The model under review builds one solid part; all positions refer to its coordinate system, in mm. A direction names the side the tool comes from. Round coordinates to 2 decimals unless told otherwise and drop trailing zeros. Order: outer loops, then holes, each group sorted by start corner. A loop starts at its lowest first (then second) coordinate and runs counter-clockwise, first axis right, second up. Notation, with made-up numbers: (-12.5, -20.5) - (38.5, -20.5) arc R25 ccw to (38.5, 4.5) - close; hole circle Ø10 at (5.5, 0). An arc over 180 degrees is marked (long way). One line per question, with ' | ' between items. Start each with the question number.
Item 1: Add section B-B on x = -138.5. State the section outline as (y, z) points, and give its area (3 significant figures).
Item 2: Insertion check: pin 1 Ø2 at (y, z) = (-5.5, -7) entering from -X; pin 2 Ø3 at (x, y) = (-75, -6.5) entering from +Z; pin 3 Ø2 at (x, z) = (91, -5) entering from -Y; pin 4 Ø1.1 at (x, y) = (177.5, -3) entering from +Z. Each pin has a flat end and moves straight along its axis. Give the tip position at first contact, or say it passes through.
Item 3: Add section A-A on x = -46.5. State the section outline as (y, z) points, and give its area (3 significant figures).
Item 4: Draft analysis for pull direction X (two halves, no side actions). For faces 1 (the face through (-2, -5, -22.777)), 2 (the face through (130.237, -5.41, -3.638)), 3 (the face through (172.41, -5.41, -3.82)), state which applies: +X half, -X half, draft (parallel to the pull), parting line (faces both ways), or undercut.
Item 5: For L1, parallel to Z at x = -57.5, y = -1; L2, parallel to Z at x = 127.5, y = -1, list the stretches that pass through material, from the lowest coordinate up. Write a range as [from, to].
Item 6: Tool access review of faces 4 (the face through (177.929, -5, -17)), 5 (the face through (164, -5.4, -3.6)): name each direction out of +Z, -Z, +X, -X, +Y, -Y from which nothing blocks a thin tool from reaching the whole face with its end or side.
from build123d import *

# Parameters (mm, degrees)
F1_DEPTH = 10.9728


with BuildPart() as f1:
    # F0 (on Front) → F1 (new body)
    with BuildSketch(Plane.XZ):
        Polygon((-177.6711943626, -10.0771774247), (-177.6711943626, -22.7771774247), (177.9288056374, -22.7771774247), (177.9288056374, -10.0771774247), (176.5609765906, -10.0771774247), (159.6928365906, -10.0771774247), (159.6916056374, -10.0771774247), (142.8246965906, -10.0771774247), (142.8234656374, -10.0771774247), (125.9565565906, -10.0771774247), (125.9553256374, -10.0771774247), (109.0884165906, -10.0771774247), (109.0871856374, -10.0771774247), (92.2202765906, -10.0771774247), (92.2190456374, -10.0771774247), (75.3521365906, -10.0771774247), (75.3509056374, -10.0771774247), (58.4839965906, -10.0771774247), (58.4827656374, -10.0771774247), (41.6158565906, -10.0771774247), (41.6146256374, -10.0771774247), (24.7477165906, -10.0771774247), (24.7464856374, -10.0771774247), (7.8795765906, -10.0771774247), (7.8783456374, -10.0771774247), (-8.9885634094, -10.0771774247), (-8.9897943626, -10.0771774247), (-25.8567034094, -10.0771774247), (-25.8579343626, -10.0771774247), (-42.7248434094, -10.0771774247), (-42.7260743626, -10.0771774247), (-59.5929834094, -10.0771774247), (-59.5942143626, -10.0771774247), (-76.4611234094, -10.0771774247), (-76.4623543626, -10.0771774247), (-93.3292634094, -10.0771774247), (-93.3304943626, -10.0771774247), (-110.1974034094, -10.0771774247), (-110.1986343626, -10.0771774247), (-127.0655434094, -10.0771774247), (-127.0667743626, -10.0771774247), (-143.9336834094, -10.0771774247), (-143.9349143626, -10.0771774247), (-160.8018234094, -10.0771774247), (-160.8030543626, -10.0771774247), align=None)
        Polygon((-169.2260503769, 2.6228225753), (-177.6711943626, -10.0771774247), (-160.8030543626, -10.0771774247), (-160.8024381229, -10.0762507093), align=None)
        Polygon((-160.8024381229, -10.0762507093), (-160.8030543626, -10.0771774247), (-160.8018234094, -10.0771774247), align=None)
        Polygon((159.6928365906, -10.0771774247), (176.5609765906, -10.0771774247), (168.1367496231, 2.6228225753), (159.6922218771, -10.0762507093), align=None)
        Polygon((-160.8024381229, -10.0762507093), (-160.8018234094, -10.0771774247), (-143.9349143626, -10.0771774247), (-143.9342981229, -10.0762507093), (-152.3579103769, 2.6228225753), align=None)
        Polygon((159.6916056374, -10.0771774247), (159.6928365906, -10.0771774247), (159.6922218771, -10.0762507093), align=None)
        Polygon((-143.9342981229, -10.0762507093), (-143.9349143626, -10.0771774247), (-143.9336834094, -10.0771774247), align=None)
        Polygon((142.8246965906, -10.0771774247), (159.6916056374, -10.0771774247), (159.6922218771, -10.0762507093), (151.2686096231, 2.6228225753), (142.8240818771, -10.0762507093), align=None)
        Polygon((-143.9342981229, -10.0762507093), (-143.9336834094, -10.0771774247), (-127.0667743626, -10.0771774247), (-127.0661581229, -10.0762507093), (-135.4897703769, 2.6228225753), align=None)
        Polygon((142.8234656374, -10.0771774247), (142.8246965906, -10.0771774247), (142.8240818771, -10.0762507093), align=None)
        Polygon((-127.0661581229, -10.0762507093), (-127.0667743626, -10.0771774247), (-127.0655434094, -10.0771774247), align=None)
        Polygon((125.9565565906, -10.0771774247), (142.8234656374, -10.0771774247), (142.8240818771, -10.0762507093), (134.4004696231, 2.6228225753), (125.9559418771, -10.0762507093), align=None)
        Polygon((-127.0661581229, -10.0762507093), (-127.0655434094, -10.0771774247), (-110.1986343626, -10.0771774247), (-110.1980181229, -10.0762507093), (-118.6216303769, 2.6228225753), align=None)
        Polygon((125.9553256374, -10.0771774247), (125.9565565906, -10.0771774247), (125.9559418771, -10.0762507093), align=None)
        Polygon((-110.1980181229, -10.0762507093), (-110.1986343626, -10.0771774247), (-110.1974034094, -10.0771774247), align=None)
        Polygon((109.0884165906, -10.0771774247), (125.9553256374, -10.0771774247), (125.9559418771, -10.0762507093), (117.5323296231, 2.6228225753), (109.0878018771, -10.0762507093), align=None)
        Polygon((-110.1980181229, -10.0762507093), (-110.1974034094, -10.0771774247), (-93.3304943626, -10.0771774247), (-93.3298781229, -10.0762507093), (-101.7534903769, 2.6228225753), align=None)
        Polygon((109.0871856374, -10.0771774247), (109.0884165906, -10.0771774247), (109.0878018771, -10.0762507093), align=None)
        Polygon((-93.3298781229, -10.0762507093), (-93.3304943626, -10.0771774247), (-93.3292634094, -10.0771774247), align=None)
        Polygon((92.2202765906, -10.0771774247), (109.0871856374, -10.0771774247), (109.0878018771, -10.0762507093), (100.6641896231, 2.6228225753), (92.2196618771, -10.0762507093), align=None)
        Polygon((-93.3298781229, -10.0762507093), (-93.3292634094, -10.0771774247), (-76.4623543626, -10.0771774247), (-76.4617381229, -10.0762507093), (-84.8853503769, 2.6228225753), align=None)
        Polygon((92.2190456374, -10.0771774247), (92.2202765906, -10.0771774247), (92.2196618771, -10.0762507093), align=None)
        Polygon((-76.4617381229, -10.0762507093), (-76.4623543626, -10.0771774247), (-76.4611234094, -10.0771774247), align=None)
        Polygon((75.3521365906, -10.0771774247), (92.2190456374, -10.0771774247), (92.2196618771, -10.0762507093), (83.7960496231, 2.6228225753), (75.3515218771, -10.0762507093), align=None)
        Polygon((-76.4617381229, -10.0762507093), (-76.4611234094, -10.0771774247), (-59.5942143626, -10.0771774247), (-59.5935981229, -10.0762507093), (-68.0172103769, 2.6228225753), align=None)
        Polygon((75.3509056374, -10.0771774247), (75.3521365906, -10.0771774247), (75.3515218771, -10.0762507093), align=None)
        Polygon((-59.5935981229, -10.0762507093), (-59.5942143626, -10.0771774247), (-59.5929834094, -10.0771774247), align=None)
        Polygon((58.4839965906, -10.0771774247), (75.3509056374, -10.0771774247), (75.3515218771, -10.0762507093), (66.9279096231, 2.6228225753), (58.4833818771, -10.0762507093), align=None)
        Polygon((-59.5935981229, -10.0762507093), (-59.5929834094, -10.0771774247), (-42.7260743626, -10.0771774247), (-42.7254581229, -10.0762507093), (-51.1490703769, 2.6228225753), align=None)
        Polygon((58.4827656374, -10.0771774247), (58.4839965906, -10.0771774247), (58.4833818771, -10.0762507093), align=None)
        Polygon((-42.7254581229, -10.0762507093), (-42.7260743626, -10.0771774247), (-42.7248434094, -10.0771774247), align=None)
        Polygon((41.6158565906, -10.0771774247), (58.4827656374, -10.0771774247), (58.4833818771, -10.0762507093), (50.0597696231, 2.6228225753), (41.6152418771, -10.0762507093), align=None)
        Polygon((-42.7254581229, -10.0762507093), (-42.7248434094, -10.0771774247), (-25.8579343626, -10.0771774247), (-25.8573181229, -10.0762507093), (-34.2809303769, 2.6228225753), align=None)
        Polygon((41.6146256374, -10.0771774247), (41.6158565906, -10.0771774247), (41.6152418771, -10.0762507093), align=None)
        Polygon((-25.8573181229, -10.0762507093), (-25.8579343626, -10.0771774247), (-25.8567034094, -10.0771774247), align=None)
        Polygon((24.7477165906, -10.0771774247), (41.6146256374, -10.0771774247), (41.6152418771, -10.0762507093), (33.1916296231, 2.6228225753), (24.7471018771, -10.0762507093), align=None)
        Polygon((-25.8573181229, -10.0762507093), (-25.8567034094, -10.0771774247), (-8.9897943626, -10.0771774247), (-8.9891781229, -10.0762507093), (-17.4127903769, 2.6228225753), align=None)
        Polygon((24.7464856374, -10.0771774247), (24.7477165906, -10.0771774247), (24.7471018771, -10.0762507093), align=None)
        Polygon((-8.9891781229, -10.0762507093), (-8.9897943626, -10.0771774247), (-8.9885634094, -10.0771774247), align=None)
        Polygon((7.8795765906, -10.0771774247), (24.7464856374, -10.0771774247), (24.7471018771, -10.0762507093), (16.3234896231, 2.6228225753), (7.8789618771, -10.0762507093), align=None)
        Polygon((-8.9891781229, -10.0762507093), (-8.9885634094, -10.0771774247), (7.8783456374, -10.0771774247), (7.8789618771, -10.0762507093), (-0.5446503769, 2.6228225753), align=None)
        Polygon((7.8783456374, -10.0771774247), (7.8795765906, -10.0771774247), (7.8789618771, -10.0762507093), align=None)
    extrude(amount=F1_DEPTH)


solid = f1.part
Determined:
1) outline: (-10.97, -22.78) - (0, -22.78) - (0, -1.9) - (-10.97, -1.9) - close | area: 229 mm2
2) pin 1: x = -176.29 | pin 2: z = -5.62 | pin 3: through | pin 4: z = -10.08
3) outline: (-10.97, -22.78) - (0, -22.78) - (0, -4.39) - (-10.97, -4.39) - close | area: 202 mm2
4) face 1: draft | face 2: undercut | face 3: +X half
5) L1: [-22.78, -6.93] | L2: [-22.78, -7.75]
6) face 4: +Z, -Z, +X, +Y, -Y | face 5: +Z, +Y, -Y
